from build123d import *

# Parameters (mm, degrees)
REVOLVE1_ANGLE            = 45
CUT_EXTRUDE1_DEPTH        = 28.647117169
CUT_EXTRUDE1_DEPTH_BACK   = 28.647117169
CUT_EXTRUDE4_REACH        = 29.998
CUT_EXTRUDE4_START_RADIUS = 14.22
CUT_EXTRUDE4_END_RADIUS   = 14.22
CUT_EXTRUDE5_DEPTH        = 26.992100662
CUT_EXTRUDE5_DEPTH_BACK   = 26.992100662
SKETCH9_R                 = 2.6035


with BuildPart() as part:
    # Sketch1 → Revolve1 (revolve, symmetric)
    with BuildSketch(Plane(origin=(0, 0, 0), x_dir=(0, 0, -1), z_dir=(1, 0, 0))) as revolve1_sk:
        with BuildLine():
            Line((-14.217802221, 0.25), (-19.048359509, 0.25))
            ThreePointArc((-19.048359509, 0.25), (-14.676690222, 12.144845166), (-3.81, 18.66511184))
            Line((-3.81, 18.66511184), (-3.81, 13.700083941))
            ThreePointArc((-3.81, 13.700083941), (-11.246181696, 8.70240181), (-14.217802221, 0.25))
        make_face()
    revolve(axis=Axis((0, 0, 0), (0, 1, 0)), revolution_arc=REVOLVE1_ANGLE / 2)
    revolve(revolve1_sk.sketch, axis=Axis((0, 0, 0), (0, -1, 0)), revolution_arc=REVOLVE1_ANGLE / 2)

    # Sketch2 → Cut-Extrude1 (cut, two sides: drawn at the far end of the back side and taken through both)
    with BuildSketch(Plane(origin=(0, 0, 0), x_dir=(1, 0, 0), z_dir=(0, 1, 0)).offset(-CUT_EXTRUDE1_DEPTH_BACK)):
        with BuildLine():
            Line((7.289491598, -17.598389479), (1.458023877, -3.519981019))
            ThreePointArc((1.458023877, -3.519981019), (1.400077392, -3.543428184), (1.341754023, -3.5659215))
            Line((1.341754023, -3.5659215), (7.173849701, -17.645845983))
            ThreePointArc((7.173849701, -17.645845983), (7.231709577, -17.622212591), (7.289491598, -17.598389479))
        make_face()
        with BuildLine():
            Line((-7.173849701, -17.645845983), (-1.341754023, -3.5659215))
            ThreePointArc((-1.341754023, -3.5659215), (-1.400077392, -3.543428184), (-1.458023877, -3.519981019))
            Line((-1.458023877, -3.519981019), (-7.289491598, -17.598389479))
            ThreePointArc((-7.289491598, -17.598389479), (-7.231709577, -17.622212591), (-7.173849701, -17.645845983))
        make_face()
    extrude(amount=CUT_EXTRUDE1_DEPTH + CUT_EXTRUDE1_DEPTH_BACK, mode=Mode.SUBTRACT)

    # Cut-Extrude4: from a sphere face, 29.998 long prism both ways, kept between that surface and its translate by the depth
    cut_extrude4_start = Location((0, 0, 0)) * Sphere(CUT_EXTRUDE4_START_RADIUS, mode=Mode.PRIVATE)
    cut_extrude4_end = Location((0, 0.145802388, 0.351998102)) * Sphere(CUT_EXTRUDE4_END_RADIUS, mode=Mode.PRIVATE)
    # Sketch8 → Cut-Extrude4 (cut, from a surface)
    with BuildSketch(Plane(origin=(0, 0, 0), x_dir=(-1, 0, 0), z_dir=(0, 0.3826834323650899, 0.9238795325112868)), mode=Mode.PRIVATE) as cut_extrude4_sk1:
        Polygon((0.887753405, -0.619026887), (0.968782051, -0.619026887), (0.968782051, 2.458280805), (1.481666667, 2.458280805), (1.481666667, 2.914178241), (0.968782051, 2.914178241), (0.968782051, 3.939947472), (0.569871795, 3.939947472), (0.569871795, 2.914178241), (-1.538653846, 2.914178241), align=None)
        Polygon((0.569871795, 2.458280805), (0.569871795, 0.5278401), (-0.755080128, 2.458280805), align=None, mode=Mode.SUBTRACT)
    cut_extrude4_tool1 = extrude(cut_extrude4_sk1.sketch, amount=CUT_EXTRUDE4_REACH, both=True, mode=Mode.PRIVATE)
    add(((cut_extrude4_tool1 - cut_extrude4_start) & cut_extrude4_end).solids().sort_by_distance((-0.928268, 5.918875, 12.814738))[0], mode=Mode.SUBTRACT)

    # Sketch9 → Cut-Extrude5 (cut, two sides: drawn at the far end of the back side and taken through both)
    with BuildSketch(Plane(origin=(2.950125281, 18.858537854, 18.626357959), x_dir=(-0.8917235779063104, -0.23968096505674769, 0.3839037582460406), z_dir=(-0.1106158710412275, -0.7071067811865475, -0.6984011233337121)).offset(-CUT_EXTRUDE5_DEPTH_BACK)):
        with Locations(Location((0, 0, 0), (0, 0, 116.203724747))):
            Circle(SKETCH9_R)
    extrude(amount=CUT_EXTRUDE5_DEPTH + CUT_EXTRUDE5_DEPTH_BACK, mode=Mode.SUBTRACT)


solid = part.part
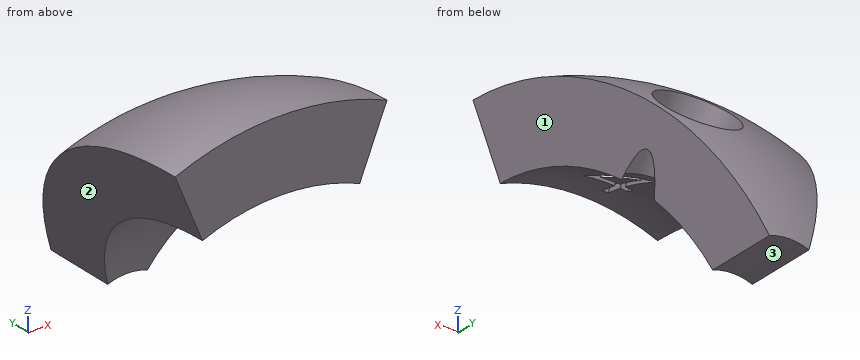
Here's how the part is built. I have some questions about the finished solid (model axes, mm). Face numbers are marked on the shaded views. Coordinates: 2 decimals unless noted, no trailing zeros. Write each loop counter-clockwise with the first axis right and the second up, starting at its lowest first coordinate (ties: lowest second). Pieces come first, ordered by that corner, then holes. Notation, with made-up numbers: (-26.75, 78) - (32.25, 78) arc R9 ccw to (32.25, 92) - close; hole circle Ø4 at (13.5, 12.25). An arc over 180 degrees is marked (long way). Use one line per item in the form item = value.
1) Thinking about a two-plate mould opening in X: for the marked faces 1, 2 and 3, which applies, released by +X, released by -X, zero draft, split by the parting line, or undercut?
Solved:
face_1 = released by +X
face_2 = released by -X
face_3 = undercut
2) I need wall thicknesses on line 1 (X direction, y = 12.5, z = 13); line 2 (Z direction, x = -5, y = 1.25); line 3 (Z direction, x = -5.5, y = 5.5). Which ranges of each line are inside material? Lowest first, please.
Solved:
line_1 = -5.25 to -0.57, 4.58 to 5.25
line_2 = 13.25 to 18.34
line_3 = 13.6 to 17.39
3) Suppose I cut it at B-B, the plane z = 7.5. Write out the boundary of the cut face in (x, y).
Solved:
outline = (-2.97, 11.71) arc R12.08 cw to (2.97, 11.71) - (2.97, 17.26) arc R17.51 ccw to (-2.97, 17.26) - close
4) Suppose I cut it at A-A, the plane x = -2. Write out the boundary of the cut face in (y, z).
Solved:
outline = (0.25, 14.08) arc R14.08 cw to (13.1, 5.16) - (18.23, 5.16) arc R18.94 ccw to (0.25, 18.94) - close
5) I'm going to push flat-ended pins straight in: P1, Ø1.5, axis at x = 5.5, z = 8.5, coming from the -Y side; P2, Ø4, axis at y = 16, z = 9, coming from the -X side; P3, Ø1, axis at x = -4.5, y = 13.5, coming from the -Z side; P4, Ø0.7, axis at y = 5, z = 13.5, coming from the +X side. Where does each tip first touch, or does it pass through?
Solved:
P1 = through
P2 = -4.33
P3 = 9.98
P4 = 5.6
